from build123d import *

# Parameters (mm, degrees)
F4_DEPTH  = 12
F6_DEPTH  = 10.4
F8_DEPTH  = 2.4
F10_DEPTH = 0.4
F12_DEPTH = 0.8


with BuildPart() as f4:
    # F3 (on Top) → F4 (new body)
    with BuildSketch(Plane.XY):
        Polygon((-28, -23.0940107676), (28, -23.0940107676), (34, -12.7017059222), (6, 35.7957166898), (-6, 35.7957166898), (-34, -12.7017059222), align=None)
    extrude(amount=F4_DEPTH)

    # F5 (on face) → F6 (cut)
    with BuildSketch(Plane.XY.offset(12)):
        Polygon((32.1524791386, -12.7017059222), (5.0762395693, 34.1957166898), (-5.0762395693, 34.1957166898), (-32.1524791386, -12.7017059222), (-27.0762395693, -21.4940107676), (27.0762395693, -21.4940107676), align=None)
    extrude(amount=-F6_DEPTH, mode=Mode.SUBTRACT)

    # F7 (on face) → F8 (join)
    with BuildSketch(Plane.XY.offset(1.6)):
        Polygon((-5, -2.8867513459), (5, -2.8867513459), (0, 5.7735026919), align=None)
    extrude(amount=F8_DEPTH)

    # F9 (on face) → F10 (join)
    with BuildSketch(Plane.XY.offset(1.6)):
        Polygon((0, 25.4034118443), (-5.0762395693, 34.1957166898), (-32.1524791386, -12.7017059222), (-27.0762395693, -21.4940107676), (-5.6666666667, 15.5884572681), align=None)
        Polygon((16.3333333333, -2.8867513459), (0, 25.4034118443), (-5.6666666667, 15.5884572681), (0, 5.7735026919), (5, -2.8867513459), align=None)
    extrude(amount=F10_DEPTH)

    # F11 (on face) → F12 (join)
    with BuildSketch(Plane.XY.offset(1.6)):
        Polygon((-10.6666666667, -12.7017059222), (32.1524791386, -12.7017059222), (5.0762395693, 34.1957166898), (-5.0762395693, 34.1957166898), (16.3333333333, -2.8867513459), (-5, -2.8867513459), align=None)
    extrude(amount=F12_DEPTH)


solid = f4.part
CAD build for the part. Positions are in the model's coordinates, mm. A direction names the side the tool comes from. Round coordinates to 2 decimals unless told otherwise and drop trailing zeros. Loops run counter-clockwise (first coordinate to the right, second up) from the corner with the lowest first, then second, coordinate; pieces in that order, holes last. Notation, with made-up numbers: M 37.5,49.25 L 55.5,49.25 A23 cw 55.5,70.25 Z; hole C 28,28.25 d2. An arc over 180 degrees is marked long. One line per question, with ' | ' between items. Start each with the question number.
Item 1: Cut at C-C, the plane x = -12. Write the cut outline in (y, z), plus the area to 3 significant figures.
Item 2: Wall check: line 1 (Y direction, x = -5, z = 7); line 2 (Z direction, x = 2, y = 25.5); line 3 (Z direction, x = -26, y = -12.5). Give the ranges that are in metal, low to high.
Item 3: Cut at B-B, the plane y = 10. Write the cut outline in (x, z), plus the area to 3 significant figures.
Item 4: Cut at A-A, the plane z = 6.5. Write the cut outline in (x, y), plus the area to 3 significant figures.
Item 5: Two-plate mould, pull along X, no slides. Class faces 1 (the flat face through (20.2, 11.2, 5.9)), 2 (the flat face through (0, -23.094, 6)), 3 (the flat face through (-19.8, 11.89, 5.92)), 4 (the flat face through (-2, -14, 1.6)): pulls with the +X half, pulls with the -X half, needs draft (parallel to the pull), parting line crosses it, or undercut.
Item 6: Cut at D-D, the plane x = 23. Write the cut outline in (y, z).
Item 7: Pin check, flat tips, straight feed: pin 1 Ø4.5 at (x, y) = (0.5, 3) entering from +Z; pin 2 Ø3 at (x, z) = (15.5, 3) entering from +Y; pin 3 Ø1.5 at (y, z) = (-13.5, 6.5) entering from +X. Stop position of each tip, or through.
Item 8: Which spindle directions (+Z, -Z, +X, -X, +Y, -Y) get a long thin tool onto all of the face, cutting with end or side? Do faces 5 (the flat face through (0, 0, 0)), 6 (the flat face through (-18.42, 11.08, 7.07)). Say none if no direction does.
Responses:
1) outline: M -23.09,0 L 25.4,0 L 25.4,12 L 22.2,12 L 22.2,2 L 4.62,2 L 4.62,1.6 L -21.49,1.6 L -21.49,12 L -23.09,12 Z | area: 135 mm²
2) line 1: y = -23.09 to -21.49, 34.2 to 35.8 | line 2: z = 0 to 2.4 | line 3: z = 0 to 2
3) outline: M -20.89,0 L 20.89,0 L 20.89,12 L 19.05,12 L 19.05,2.4 L 8.89,2.4 L 8.89,2 L -2.44,2 L -2.44,1.6 L -8.89,1.6 L -8.89,2 L -19.05,2 L -19.05,12 L -20.89,12 Z | area: 122 mm²
4) outline: M -34,-12.7 L -28,-23.09 L 28,-23.09 L 34,-12.7 L 6,35.8 L -6,35.8 Z; hole M -32.15,-12.7 L -27.08,-21.49 L 27.08,-21.49 L 32.15,-12.7 L 5.08,34.2 L -5.08,34.2 Z | area: 318 mm²
5) face 1: pulls with the +X half | face 2: needs draft | face 3: pulls with the -X half | face 4: undercut
6) outline: M -23.09,0 L 6.35,0 L 6.35,12 L 3.15,12 L 3.15,2.4 L -12.7,2.4 L -12.7,1.6 L -21.49,1.6 L -21.49,12 L -23.09,12 Z
7) pin 1: stops at z = 4 | pin 2: stops at y = 21.94 | pin 3: stops at x = 33.97
8) face 5: -Z, +X, -X, +Y, -Y | face 6: +Z
